```python
from build123d import *

# Parameters (mm, degrees)
EXTRUDE_1_DEPTH     = 37
SHELL_1_T           = -3
SKETCH_2_R          = 1.1
CUT_EXTRUDE_1_DEPTH = 30
SKETCH_3_R          = 6.5
CUT_EXTRUDE_2_DEPTH = 5
SKETCH_4_R          = 1.4
CUT_EXTRUDE_3_DEPTH = 5


with BuildPart() as part:
    # ｽｹｯﾁ1 → ﾎﾞｽ - 押し出し1 (new body)
    with BuildSketch(Plane.XY):
        Polygon((0, 0), (32, 0), (32, 28.179721765), align=None)
    extrude(amount=EXTRUDE_1_DEPTH)

    # ｼｪﾙ1
    shell_1_openings = [part.faces().sort_by_distance(p)[0] for p in [
        (16, 14.089860882, 18.5),
    ]]
    offset(amount=SHELL_1_T, openings=shell_1_openings, kind=Kind.INTERSECTION)

    # ｽｹｯﾁ2 → ｶｯﾄ - 押し出し1 (cut)
    with BuildSketch(Plane.XZ):
        with Locations(Location((26.57, 10.5, 0), (0, 0, 270))):
            Circle(SKETCH_2_R)
        with Locations(Location((5.57, 10.5, 0), (0, 0, 270))):
            Circle(SKETCH_2_R)
        with Locations(Location((5.57, 31.5, 0), (0, 0, 270))):
            Circle(SKETCH_2_R)
        with Locations(Location((26.57, 31.5, 0), (0, 0, 270))):
            Circle(SKETCH_2_R)
    extrude(amount=-CUT_EXTRUDE_1_DEPTH, mode=Mode.SUBTRACT)

    # ｽｹｯﾁ3 → ｶｯﾄ - 押し出し2 (cut)
    with BuildSketch(Plane.XZ):
        with Locations(Location((16.07, 10.5, 0), (0, 0, 270))):
            Circle(SKETCH_3_R)
    extrude(amount=-CUT_EXTRUDE_2_DEPTH, mode=Mode.SUBTRACT)

    # ｽｹｯﾁ4 → ｶｯﾄ - 押し出し3 (cut)
    with BuildSketch(Plane(origin=(32, 0, 0), x_dir=(0, 0, -1), z_dir=(1, 0, 0))):
        with Locations((-6, 22.679721765)):
            Circle(SKETCH_4_R)
        with Locations((-31, 22.679721765)):
            Circle(SKETCH_4_R)
        with Locations((-31, 7.679721765)):
            Circle(SKETCH_4_R)
        with Locations((-6, 7.679721765)):
            Circle(SKETCH_4_R)
    extrude(amount=-CUT_EXTRUDE_3_DEPTH, mode=Mode.SUBTRACT)


solid = part.part
```
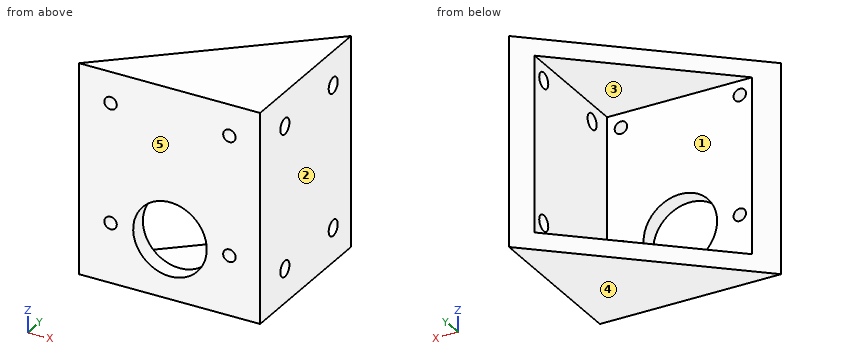
Can you work these out from the model? Positions are in its coordinate system, mm. Face numbers are marked on the shaded views. A direction names the side the tool comes from. Coordinates: 2 decimals unless noted, no trailing zeros. Loops run counter-clockwise (first coordinate to the right, second up) from the corner with the lowest first, then second, coordinate; pieces in that order, holes last. Notation, with made-up numbers: M 26.5,38 L 68.5,38 A23 cw 68.5,61 Z; hole C 69,80.5 d2. An arc over 180 degrees is marked long. Put each result on its own line as item: value. Start each with the question number.
(1) Which directions (+Z, -Z, +X, -X, +Y, -Y) give clear straight access to the entire face, cutting with the end or side of a thin tool? Please do the marked faces 1 and 2.
(2) I need wall thicknesses on probe 1 along Z at (x, y) = (19, 3.75); probe 2 along X at (y, z) = (1.75, 31.5); probe 3 along Y at (x, z) = (21, 19.5). Which ranges of each line are inside material? Lowest first, please.
(3) Imagine slicing it at D-D on y = 2. List the corners of the cut face in (x, z) for me.
(4) Imagine slicing it at B-B on x = 18. List the corners of the cut face in (y, z) for me, and give its area (3 significant figures).
(5) Imagine slicing it at A-A on z = 8. List the corners of the cut face in (x, y) for me.
(6) Imagine slicing it at C-C on z = 31. List the corners of the cut face in (x, y) for me.
(7) We'd pull the mould along Z, two halves only. Please class the marked faces 3, 4 and 5: +Z half, -Z half, draft (parallel to the pull), parting line (faces both ways), or undercut.
(8) Will these pins go through, and if not, where does the flat tip stop? pin 1 Ø4.5 at (y, z) = (22.68, 31) entering from +X; pin 2 Ø13 at (x, z) = (18, 11) entering from +Y; pin 3 Ø1.5 at (y, z) = (7.5, 13) entering from -X.
Worked answers:
1. face 1: -X, +Y
1. face 2: +Z, -Z, +X, +Y, -Y
2. probe 1: z = 0 to 3, 34 to 37
2. probe 2: x = 1.99 to 4.47, 6.67 to 25.47, 27.67 to 32
2. probe 3: y = 0 to 3
3. outline: M 2.27,0 L 32,0 L 32,37 L 2.27,37 Z; hole C 5.57,10.5 d2.2; hole C 5.57,31.5 d2.2; hole C 16.07,10.5 d13; hole C 26.57,10.5 d2.2; hole C 26.57,31.5 d2.2
4. outline: M 0,0 L 15.85,0 L 15.85,3 L 3,3 L 3,4.29 L 0,4.29 Z; M 0,16.71 L 3,16.71 L 3,34 L 15.85,34 L 15.85,37 L 0,37 Z
4. area: 151 mm2
5. outline: M 0,0 L 10.07,0 L 10.07,3 L 3.41,3 Z; M 22.07,0 L 32,0 L 32,28.18 L 29,25.54 L 29,3 L 22.07,3 Z
6. outline: M 0,0 L 4.59,0 L 4.59,3 L 3.41,3 Z; M 6.55,0 L 25.59,0 L 25.59,3 L 6.55,3 Z; M 27.55,0 L 32,0 L 32,6.28 L 29,6.28 L 29,3 L 27.55,3 Z; M 29,9.08 L 32,9.08 L 32,21.28 L 29,21.28 Z; M 29,24.08 L 32,24.08 L 32,28.18 L 29,25.54 Z
7. face 3: undercut
7. face 4: -Z half
7. face 5: draft
8. pin 1: stops at x = 32
8. pin 2: stops at y = 3
8. pin 3: stops at x = 29
